Autodesk Inventor part; units mm, degrees
ref_plane "YZ Plane" through (0, 0, 0) normal (1, 0, 0) x (0, 1, 0)
ref_plane "XZ Plane" through (0, 0, 0) normal (0, 1, 0) x (-1, 0, 0)
ref_plane "XY Plane" through (0, 0, 0) normal (0, 0, 1) x (1, 0, 0)
sketch "Sketch1" plane through (0, 0, 0) normal (0, 1, 0) x (-1, 0, 0)
  line L0 (0, 0) -> (215, 0)
  line L1 (215, 0) -> (215, 115)
  line L2 (215, 115) -> (0, 115)
  line L3 (0, 115) -> (0, 0)
  dimension "d0" = 215
  dimension "d1" = 115
extrude "Extrusion1" add sketch "Sketch1" along normal blind 50
sketch "Sketch2" plane through (0, 50, 0) normal (0, 1, 0) x (1, 0, 0)
  line L0 (0, 0) -> (-215, 0)
  line L1 (-215, 0) -> (-215, -115)
  line L2 (-215, -115) -> (0, -115)
  line L3 (0, -115) -> (0, 0)
  line L4 (-215, -3) -> (-187.5, -3)
  line L5 (-187.5, -3) -> (-187.5, -112)
  line L6 (-187.5, -112) -> (-215, -112)
  dimension "d4" = 27.5
  dimension "d5" = 3
  dimension "d6" = 3
extrude "Extrusion2" cut sketch "Sketch2" against normal blind 45 contours L4 L5 L6 L1
fillet "Fillet1" radius 2 10 edges at (-107.5, 50, 115) (-107.5, 0, 115) (-107.5, 50, 0) (0, 50, 57.5) (0, 0, 57.5) (0, 25, 115) (0, 25, 0) (-215, 25, 115) (-215, 0, 57.5) (-215, 25, 0)
fillet "Fillet2" radius 2 1 edges at (-187.5, 50, 57.5)
sketch "Sketch3" plane through (0, 5, 0) normal (0, 1, 0) x (1, 0, 0)
  line L0 (-215, -112) -> (-215, -3)
  line L1 (-187.5, -112) -> (-215, -112)
  line L2 (-187.5, -3) -> (-187.5, -112)
  line L3 (-215, -3) -> (-187.5, -3)
  line L4 (-212, -110) -> (-212, -38)
  line L5 (-212, -38) -> (-187.5, -38)
  line L6 (-212, -110) -> (-187.5, -110)
  point P0 (0, 0)
  dimension "d14" = 3
  dimension "d15" = 2
  dimension "d16" = 72
extrude "Extrusion3" add sketch "Sketch3" along normal blind 5 contours L6 L4 L5 L2
sketch "Sketch4" plane through (0, 10, 0) normal (0, 1, 0) x (1, 0, 0)
  line L0 (-212, -110) -> (-187.5, -110)
  line L1 (-212, -38) -> (-212, -110)
  circle A0 centre (-206, -45.5) radius 3
  circle A1 centre (-206, -55) radius 3
  circle A2 centre (-206, -64.5) radius 3
  circle A3 centre (-206, -74) radius 3
  circle A4 centre (-206, -83.5) radius 3
  circle A5 centre (-206, -93) radius 3
  circle A6 centre (-206, -102.5) radius 3
  point P0 (0, 0)
  dimension "d19" = 6
  dimension "d25" = 9.5
  dimension "d26" = 9.5
  dimension "d27" = 9.5
  dimension "d28" = 9.5
  dimension "d29" = 9.5
  dimension "d30" = 9.5
  dimension "d31" = 7.5
  dimension "d32" = 6
extrude "Extrusion4" add sketch "Sketch4" along normal blind 6
fillet "Fillet3" radius 2 3 edges at (-214.4142, 0.5858, 0.5858) (-0.5858, 0.5858, 0.5858) (-107.5, 0, 0)
properties part number "PSUUltibots"
Verification items for the finished model (mm, model axes). A direction names the side the tool comes from. Coordinates: 2 decimals unless noted, no trailing zeros. Write each loop counter-clockwise with the first axis right and the second up, starting at its lowest first coordinate (ties: lowest second). Pieces come first, ordered by that corner, then holes. Notation, with made-up numbers: (80, 39.25) -> (137, 39.25) arc R21 ccw to (137, 57.25) -> close; hole circle Ø1 at (27, 48). An arc over 180 degrees is marked (long way). One line per item, written item: value. Start each with the question number.
Q1. Cross-section at A-A on y = 14. Enter the section's corners in (x, z).
Q2. Cross-section at D-D on z = 17.5. Enter the section's corners in (x, y).
Q3. Thickness scan on L1, parallel to X at y = 33, z = 78.5; L2, parallel to Y at x = -189.5, z = 70.5. Record the ranges inside material, lowest first. Write a range as from..to.
Q4. Access from +Z, -Z, +X, -X, +Y, -Y to the whole of each face (thin tool, end or side, straight path). Record for faces 1 (the flat face through (-215, 3, 57)), 2 (the flat face through (-200, 10, 73)), 3 (the flat face through (-206, 16, 74)).
Q5. Go/stop test with flat-tipped pins: P1, Ø21.5, axis at y = 33.5, z = 63.5, coming from the -X side; P2, Ø10, axis at y = 13, z = 47, coming from the -X side; P3, Ø5, axis at x = -207, z = 46, coming from the +Y side. Record where each tip stops, or that it passes through.
Q6. Mould release check, pull along Z, two halves, no side actions. Record for faces 4 (the flat face through (-106, 25, 0)), 5 (the flat face through (0, 25, 58)), 6 (the flat face through (-109, 25, 115)), 7 (the flat face through (-206, 16, 93)): pulls with the +Z half, pulls with the -Z half, needs draft (parallel to the pull), parting line crosses it, or undercut.
Q7. Cross-section at B-B on z = 93. Enter the section's corners in (x, y).
Q8. Cross-section at C-C on y = 37. Enter the section's corners in (x, z), and give its area (3 significant figures).
Checked values:
1. outline: (-215, 2) arc R2 ccw to (-213, 0) -> (-2, 0) arc R2 ccw to (0, 2) -> (0, 113) arc R2 ccw to (-2, 115) -> (-213, 115) arc R2 ccw to (-215, 113) -> (-215, 112) -> (-187.5, 112) -> (-187.5, 3) -> (-215, 3) -> close; circle Ø6 at (-206, 45.5); circle Ø6 at (-206, 55); circle Ø6 at (-206, 64.5); circle Ø6 at (-206, 74); circle Ø6 at (-206, 83.5); circle Ø6 at (-206, 93); circle Ø6 at (-206, 102.5)
2. outline: (-215, 2) arc R2 ccw to (-213, 0) -> (-2, 0) arc R2 ccw to (0, 2) -> (0, 48) arc R2 ccw to (-2, 50) -> (-185.5, 50) arc R2 ccw to (-187.5, 48) -> (-187.5, 5) -> (-215, 5) -> close
3. L1: x = -187.5..0
3. L2: y = 0..10
4. face 1: +Z, -Z, -X, +Y, -Y
4. face 2: +Y
4. face 3: -X, +Y
5. P1: stops at x = -187.5
5. P2: stops at x = -212
5. P3: stops at y = 16
6. face 4: pulls with the -Z half
6. face 5: needs draft
6. face 6: pulls with the +Z half
6. face 7: undercut
7. outline: (-215, 2) arc R2 ccw to (-213, 0) -> (-2, 0) arc R2 ccw to (0, 2) -> (0, 48) arc R2 ccw to (-2, 50) -> (-185.5, 50) arc R2 ccw to (-187.5, 48) -> (-187.5, 10) -> (-203, 10) -> (-203, 16) -> (-209, 16) -> (-209, 10) -> (-212, 10) -> (-212, 5) -> (-215, 5) -> close
8. outline: (-215, 2) arc R2 ccw to (-213, 0) -> (-2, 0) arc R2 ccw to (0, 2) -> (0, 113) arc R2 ccw to (-2, 115) -> (-213, 115) arc R2 ccw to (-215, 113) -> (-215, 112) -> (-187.5, 112) -> (-187.5, 3) -> (-215, 3) -> close
8. area: 21,700 mm²
